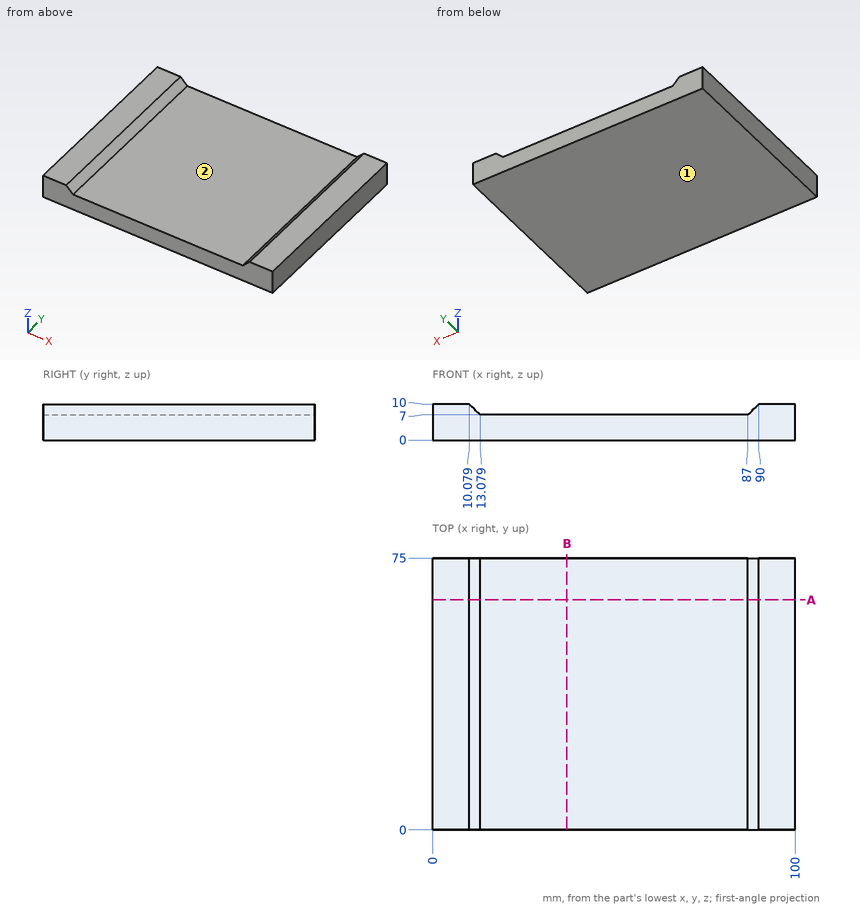
Check sheet for the drawn part. Datum: minimum x, y, z corner. Units: mm. Give positions to 0.01 mm unless a question says otherwise; leave off trailing zeros. Order: outer loops, then holes, each group sorted by start corner. A loop starts at its lowest first (then second) coordinate and runs counter-clockwise, first axis right, second up. Notation, with made-up numbers: (-12.75, 53) -> (12.25, 53) arc R12 ccw to (12.25, 59) -> close; hole circle Ø11 at (-20.75, 9.5). An arc over 180 degrees is marked (long way). Return JSON: item names as keys, results as strings.
1. Cross-section at B-B, the plane x = 37. Record the cut outline in (y, z), plus the area to 3 significant figures.
From the geometry:
{"outline": "(0, 0) -> (75, 0) -> (75, 7) -> (0, 7) -> close", "area": "525 mm^2"}
2. Go/stop test with flat-tipped pins: P1, Ø1, axis at y = 63.5, z = 6, coming from the -X side; P2, Ø4, axis at x = 47, y = 30, coming from the +Z side. Record where each tip stops, or that it passes through.
From the geometry:
{"P1": "x = 0", "P2": "z = 7"}
3. Material ranges on probe 1 along Z at (x, y) = (79, 41); probe 2 along X at (y, z) = (38.5, 7.75); probe 3 along X at (y, z) = (21, 7.5), recorded low to high. Write a range as [from, to].
From the geometry:
{"probe 1": "[0, 7]", "probe 2": "[0, 12.33], [87.75, 100]", "probe 3": "[0, 12.58], [87.5, 100]"}
4. Mould release check, pull along X, two halves, no side actions. Record for the marked faces 1 and 2: +X half, -X half, draft (parallel to the pull), parting line (faces both ways), or undercut.
From the geometry:
{"face 1": "draft", "face 2": "undercut"}
5. Cross-section at A-A, the plane y = 63.5. Record the cut outline in (x, z).
From the geometry:
{"outline": "(0, 0) -> (100, 0) -> (100, 10) -> (90, 10) -> (87, 7) -> (13.08, 7) -> (10.08, 10) -> (0, 10) -> close"}
